```python
from build123d import *

# Parameters (mm, degrees)
EXTRUDE_1_DEPTH     = 3
SKETCH_2_R          = 1.6
CUT_EXTRUDE_1_DEPTH = 62.654602424
CUT_EXTRUDE_2_DEPTH = 62.654602424
CUT_EXTRUDE_3_DEPTH = 62.654602424
FILLET_2_R          = 0.5


with BuildPart() as part:
    # 草图1 → 凸台-拉伸1 (new body)
    with BuildSketch(Plane(origin=(0, 0, 0), x_dir=(1, 0, 0), z_dir=(0, 1, 0))):
        Polygon((-55, 27.7), (-43.5, 27.7), (-33.5, 27.7), (33.5, 27.7), (43.5, 27.7), (55, 27.7), (55, -27.7), (43.5, -27.7), (33.5, -27.7), (-33.5, -27.7), (-43.5, -27.7), (-55, -27.7), align=None)
    extrude(amount=EXTRUDE_1_DEPTH)

    # 草图2 → 切除-拉伸1 (cut, through all)
    with BuildSketch(Plane(origin=(0, 3, 0), x_dir=(1, 0, 0), z_dir=(0, 1, 0))):
        with Locations(Location((0, 24.7, 0), (0, 0, 270))):
            Circle(SKETCH_2_R)
        with Locations(Location((20, 24.7, 0), (0, 0, 270))):
            Circle(SKETCH_2_R)
        with Locations(Location((20, -24.7, 0), (0, 0, 90))):
            Circle(SKETCH_2_R)
        with Locations(Location((0, -24.7, 0), (0, 0, 90))):
            Circle(SKETCH_2_R)
    extrude(amount=-CUT_EXTRUDE_1_DEPTH, mode=Mode.SUBTRACT)

    # 草图4 → 切除-拉伸2 (cut, through all)
    with BuildSketch(Plane.XZ):
        Polygon((-31.443462795, 25.668589291), (-34.443462795, 11.332567733), (-31.443462795, 15.419941133), (-28.443462795, 11.332567733), align=None)
    extrude(amount=-CUT_EXTRUDE_2_DEPTH, mode=Mode.SUBTRACT)

    # 草图5 → 切除-拉伸3 (cut, through all)
    with BuildSketch(Plane.XZ):
        Polygon((-49.924888237, 21.024053863), (-41.932272719, 21.024053863), (-45.928580478, -23.688259036), align=None)
        Polygon((-39.084223489, 7.546349568), (-32.023477439, 7.546349568), (-35.553850464, -23.688259036), align=None)
        Polygon((-24.685839388, 21.024053863), (-18.871107346, 21.024053863), (-24.685839388, -20.142850627), align=None)
        Polygon((-15.944927595, 21.024053863), (-21.778473367, -20.276047316), (-15.944927595, -20.276047316), align=None)
        Polygon((-13.685839388, -20.142850627), (-13.685839388, 21.024053863), (-7.871107346, 21.024053863), align=None)
        Polygon((-4.944927595, -20.276047316), (-4.944927595, 21.024053863), (-10.778473367, -20.276047316), align=None)
        Polygon((-2.685839388, -20.142850627), (-2.685839388, 21.024053863), (3.128892654, 21.024053863), align=None)
        Polygon((6.055072405, -20.276047316), (6.055072405, 21.024053863), (0.221526633, -20.276047316), align=None)
        Polygon((8.314160612, -20.142850627), (8.314160612, 21.024053863), (14.128892654, 21.024053863), align=None)
        Polygon((17.055072405, -20.276047316), (17.055072405, 21.024053863), (11.221526633, -20.276047316), align=None)
        Polygon((19.314160612, -20.142850627), (19.314160612, 21.024053863), (25.128892654, 21.024053863), align=None)
        Polygon((28.055072405, -20.276047316), (28.055072405, 21.024053863), (22.221526633, -20.276047316), align=None)
        Polygon((30.314160612, -20.142850627), (30.314160612, 21.024053863), (36.128892654, 21.024053863), align=None)
        Polygon((39.055072405, -20.276047316), (39.055072405, 21.024053863), (33.221526633, -20.276047316), align=None)
        Polygon((41.314160612, -20.142850627), (41.314160612, 21.024053863), (47.128892654, 21.024053863), align=None)
        Polygon((50.055072405, -20.276047316), (50.055072405, 21.024053863), (44.221526633, -20.276047316), align=None)
    extrude(amount=-CUT_EXTRUDE_3_DEPTH, mode=Mode.SUBTRACT)

    # 圆角2
    fillet_2_edges = [part.edges().sort_by_distance(p)[0] for p in [
        (-45.928580478, 1.5, -23.688259036),
        (-49.924888237, 1.5, 21.024053863),
        (-41.932272719, 1.5, 21.024053863),
        (30.314160612, 1.5, 21.024053863),
        (36.128892654, 1.5, 21.024053863),
        (30.314160612, 1.5, -20.142850627),
        (22.221526633, 1.5, -20.276047316),
        (28.055072405, 1.5, 21.024053863),
        (28.055072405, 1.5, -20.276047316),
        (19.314160612, 1.5, 21.024053863),
        (25.128892654, 1.5, 21.024053863),
        (19.314160612, 1.5, -20.142850627),
        (11.221526633, 1.5, -20.276047316),
        (17.055072405, 1.5, 21.024053863),
        (17.055072405, 1.5, -20.276047316),
        (44.221526633, 1.5, -20.276047316),
        (50.055072405, 1.5, 21.024053863),
        (50.055072405, 1.5, -20.276047316),
        (41.314160612, 1.5, 21.024053863),
        (47.128892654, 1.5, 21.024053863),
        (41.314160612, 1.5, -20.142850627),
        (33.221526633, 1.5, -20.276047316),
        (39.055072405, 1.5, 21.024053863),
        (39.055072405, 1.5, -20.276047316),
        (-13.685839388, 1.5, 21.024053863),
        (-7.871107346, 1.5, 21.024053863),
        (-13.685839388, 1.5, -20.142850627),
        (-15.944927595, 1.5, 21.024053863),
        (-15.944927595, 1.5, -20.276047316),
        (-21.778473367, 1.5, -20.276047316),
        (-24.685839388, 1.5, -20.142850627),
        (-24.685839388, 1.5, 21.024053863),
        (-18.871107346, 1.5, 21.024053863),
        (-35.553850464, 1.5, -23.688259036),
        (-39.084223489, 1.5, 7.546349568),
        (-32.023477439, 1.5, 7.546349568),
        (8.314160612, 1.5, 21.024053863),
        (14.128892654, 1.5, 21.024053863),
        (8.314160612, 1.5, -20.142850627),
        (0.221526633, 1.5, -20.276047316),
        (6.055072405, 1.5, 21.024053863),
        (6.055072405, 1.5, -20.276047316),
        (-2.685839388, 1.5, 21.024053863),
        (3.128892654, 1.5, 21.024053863),
        (-2.685839388, 1.5, -20.142850627),
        (-10.778473367, 1.5, -20.276047316),
        (-4.944927595, 1.5, 21.024053863),
        (-4.944927595, 1.5, -20.276047316),
        (-55, 1.5, 27.7),
        (-55, 1.5, -27.7),
        (55, 1.5, -27.7),
        (55, 1.5, 27.7),
        (-31.443462795, 1.5, 25.668589291),
        (-28.443462795, 1.5, 11.332567733),
        (-31.443462795, 1.5, 15.419941133),
        (-34.443462795, 1.5, 11.332567733),
    ]]
    fillet(fillet_2_edges, radius=FILLET_2_R)


solid = part.part
```
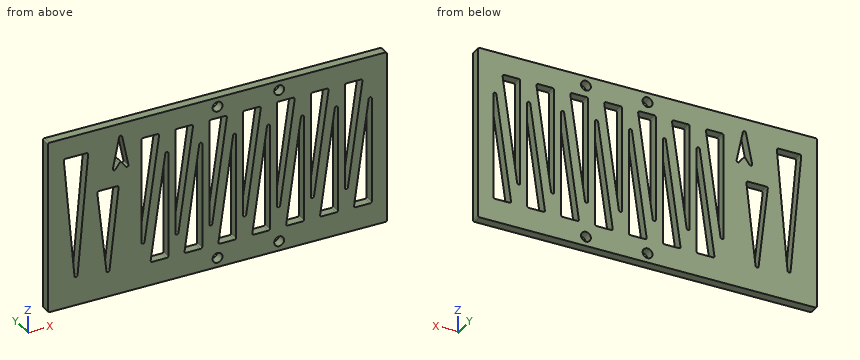
Work out the finished part from the listing and answer in its coordinate system (mm). Round coordinates to 2 decimals unless told otherwise and drop trailing zeros. Write each loop counter-clockwise with the first axis right and the second up, starting at its lowest first coordinate (ties: lowest second). Pieces come first, ordered by that corner, then holes. Notation, with made-up numbers: (18, 19) - (71, 19) arc R24 cw to (71, 32) - close; hole circle Ø7 at (69.25, 1). An arc over 180 degrees is marked (long way). Return JSON: item names as keys, results as strings. Group by question number.
Q1. The part is cut by section B-B on x = -47.5. Write down the section's boundary in (y, z), then the cut area to 3 significant figures.
Q2. The part is cut by section C-C on y = 2.55. Count the separate pieces of the cut face and the enclosed holes in it, then the cut area to 3 significant figures.
Q3. The part is cut by section A-A on z = -24.7. Write down the section's boundary in (x, y).
Q4. Find the intervals of material crossed by L1, parallel to X at y = 1.95, z = -24.7; L2, parallel to Z at x = 38.5, y = 2.3; L3, parallel to X at y = 2.8, z = 23, in increasing order.
Q5. This flat-tipped pin is pushed along its axis until it touches: pin 1 Ø1 at (x, z) = (-39.5, 15.5) entering from -Y. Where does it stop, or does it pass through?
Solved:
{
 "1": {"outline": "(0, -27.7) - (3, -27.7) - (3, -6.11) - (0, -6.11) - close; (0, 21.02) - (3, 21.02) - (3, 27.7) - (0, 27.7) - close", "area": "84.8 mm²"},
 "2": {"separate pieces": "1", "enclosed holes": "21", "area": "4,110 mm²"},
 "3": {"outline": "(-55, 0) - (-1.6, 0) - (-1.6, 3) - (-55, 3) - close; (1.6, 0) - (18.4, 0) - (18.4, 3) - (1.6, 3) - close; (21.6, 0) - (55, 0) - (55, 3) - (21.6, 3) - close"},
 "4": {"L1": "-55 to -1.6, 1.6 to 18.4, 21.6 to 55", "L2": "-27.7 to -20.28, 14.41 to 27.7", "L3": "-55 to -32, -30.89 to 55"},
 "5": {"pin 1": "y = 0"}
}
